The figure shows three views and two pictorial views of one solid part (mm, origin at its lowest corner). Answer the questions. A direction names the side the tool comes from. Coordinates: 2 decimals unless noted, no trailing zeros. Order: outer loops, then holes, each group sorted by start corner. A loop starts at its lowest first (then second) coordinate and runs counter-clockwise, first axis right, second up. Notation, with made-up numbers: (11.5, 58.25) -> (33.5, 58.25) arc R7 ccw to (33.5, 64.25) -> close; hole circle Ø6 at (-27.75, 27.25). An arc over 180 degrees is marked (long way). Write item = value, one per line.
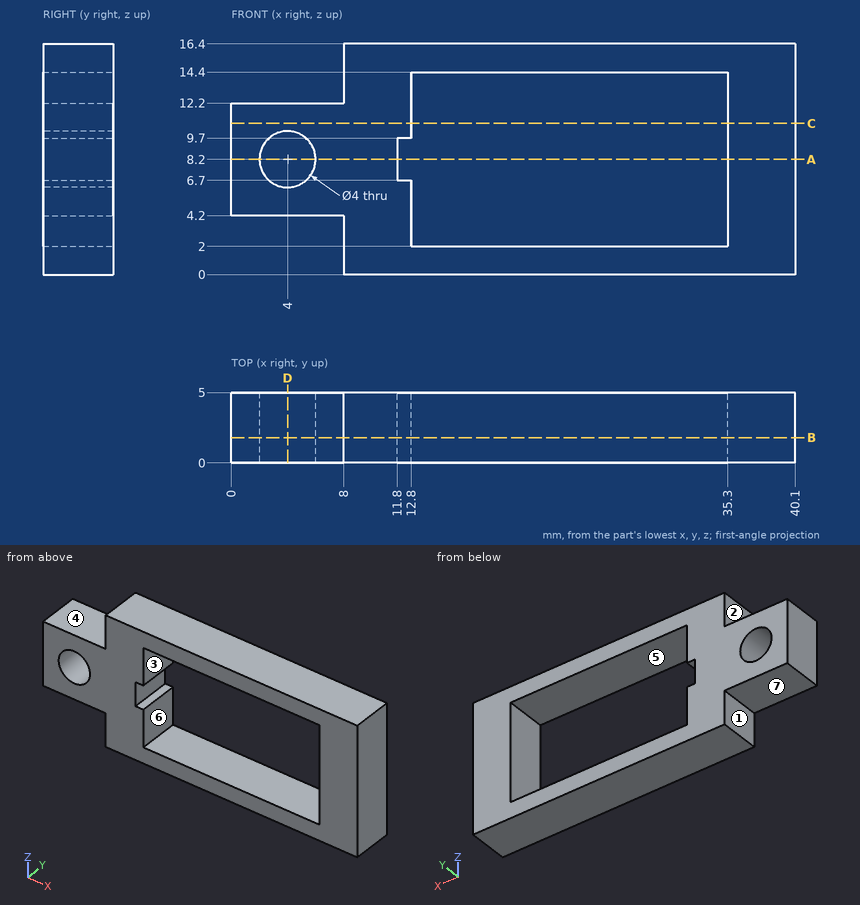
Q1. Find the intervals of material crossed by line 1 along Z through (x, y) = (4, 1.8); line 2 along X through (y, z) = (2.2, 2.75); line 3 along X through (y, z) = (3.2, 15.25), in increasing order.
The answers:
line_1 = 4.2 to 6.2, 10.2 to 12.2
line_2 = 8 to 12.8, 35.3 to 40.1
line_3 = 8 to 40.1
Q2. A tool of negligible diameter and unlimited length cuts with its end or side. For the marked faces 1, 2 and 3, from which of +Z, -Z, +X, -X, +Y, -Y can it reach the whole face along a straight path? Write none if from no direction.
The answers:
face_1 = -Z, -X, +Y, -Y
face_2 = +Z, -X, +Y, -Y
face_3 = +Y, -Y
Q3. Section D-D, the plane x = 4 is taken. Give the vertices of the cut face in (y, z), plus the area to 3 significant figures.
The answers:
outline = (0, 4.2) -> (5, 4.2) -> (5, 6.2) -> (0, 6.2) -> close; (0, 10.2) -> (5, 10.2) -> (5, 12.2) -> (0, 12.2) -> close
area = 20.0 mm2
Q4. Section A-A, the plane z = 8.2 is taken. Give the vertices of the cut face in (x, y).
The answers:
outline = (0, 0) -> (2, 0) -> (2, 5) -> (0, 5) -> close; (6, 0) -> (11.8, 0) -> (11.8, 5) -> (6, 5) -> close; (35.3, 0) -> (40.1, 0) -> (40.1, 5) -> (35.3, 5) -> close
Q5. Section B-B, the plane y = 1.8 is taken. Give the vertices of the cut face in (x, z).
The answers:
outline = (0, 4.2) -> (8, 4.2) -> (8, 0) -> (40.1, 0) -> (40.1, 16.4) -> (8, 16.4) -> (8, 12.2) -> (0, 12.2) -> close; hole circle Ø4 at (4, 8.2); hole (11.8, 6.7) -> (12.8, 6.7) -> (12.8, 2) -> (35.3, 2) -> (35.3, 14.4) -> (12.8, 14.4) -> (12.8, 9.7) -> (11.8, 9.7) -> close
Q6. Each of these flat-tipped pins is pushed along its axis until it touches: pin 1 Ø2.5 at (x, y) = (4, 1.5) entering from -Z; pin 2 Ø2 at (y, z) = (2, 13.5) entering from -X; pin 3 Ø2.5 at (x, y) = (5.5, 3.5) entering from +Z. Where does it stop, or does it pass through?
The answers:
pin_1 = 4.2
pin_2 = 8
pin_3 = 12.2
Q7. The mould has two halves that part along Z. Classify the marked faces 4, 5, 6 and 7: released by +Z, released by -Z, zero draft, split by the parting line, or undercut.
The answers:
face_4 = released by +Z
face_5 = undercut
face_6 = undercut
face_7 = released by -Z
Q8. Section C-C, the plane z = 10.75 is taken. Give the vertices of the cut face in (x, y).
The answers:
outline = (0, 0) -> (12.8, 0) -> (12.8, 5) -> (0, 5) -> close; (35.3, 0) -> (40.1, 0) -> (40.1, 5) -> (35.3, 5) -> close
